Input: part model. Units: mm. Frame: model coordinates. A direction names the side the tool comes from. Coordinates: 2 decimals unless noted, no trailing zeros. Loops run counter-clockwise (first coordinate to the right, second up) from the corner with the lowest first, then second, coordinate; pieces in that order, holes last.
(1) Section C-C, the plane y = 21. Return loops of the section in (x, z), then the cut area to 3 significant figures.
(2) Set-up query: faces 5 (the face through (0.75, 43.7, -0.1)), 6 (the face through (1, 44, -17)), 7 (the face through (-1.2, 47.5, 0.1)). Return all of +Z, -Z, +X, -X, +Y, -Y with unobstructed straight access to the full face (end or side cutting, diameter ignored); none if empty.
(3) Section B-B, the plane z = -10.5. Return loops of the section in (x, y).
(4) Section A-A, the plane z = 0. Return loops of the section in (x, y), then the cut area to 3 significant figures.
(5) Contact query for flat-ended pins moving along their axis: P1, Ø12, axis at y = 27, z = -19.5, coming from the -X side; P2, Ø1.1, axis at x = 1, z = 8, coming from the +Y side; P3, Ø0.5, axis at x = -1.5, z = 2, coming from the +Y side; P4, Ø0.8, axis at x = 1, z = -1, coming from the +Y side. Output: stop coordinate, or through.
(6) Mould query, pull axis Z, two halves, no side actions, for faces 1 (the face through (0, -1, -28.25)), 2 (the face through (1.3, 47.5, 0.1)), 3 (the face through (-0.75, 43.7, -0.1)), 4 (the face through (1, 44, 16)). Classes: released by +Z, released by -Z, zero draft, split by the parting line, or undercut.
(7) Line query: L1, parallel to Z at x = 0.3, y = 23; L2, parallel to Z at x = -1.05, y = 31; L3, parallel to Y at x = 0.9, z = 8. Output: solid intervals per line, ascending.
```python
from build123d import *

# Parameters (mm, degrees)
F1_DEPTH      = 1.75
F2_W          = 1.5
F2_H          = 55
F3_DEPTH      = 43.25
F3_DEPTH_BACK = 58.6


with BuildPart() as f1:
    # F0 (on Right) → F1 (new body, symmetric)
    with BuildSketch(Plane.YZ):
        Polygon((-42.75, -27), (-42.75, 27), (-41.75, 27), (-41.75, 28.25), (-44, 28.25), (-44, -28.25), (-41.75, -28.25), (-41.75, -27), align=None)
        Polygon((-41.75, 27), (-42.75, 27), (-42.75, -27), (-41.75, -27), (-41.75, -26), (-41.75, 26), align=None)
        Polygon((-41.75, 28.25), (-41.75, 27), (42.75, 27), (42.75, -27), (-41.75, -27), (-41.75, -28.25), (44, -28.25), (44, -5), (44, -3.5), (44, 3.5), (44, 5), (44, 28.25), align=None)
        with BuildLine():
            ThreePointArc((44, -5), (49, 0), (44, 5))
            Line((44, 5), (44, 3.5))
            ThreePointArc((44, 3.5), (47.5, 0), (44, -3.5))
            Line((44, -3.5), (44, -5))
        make_face()
    extrude(amount=F1_DEPTH, both=True)

    # F2 (on Front) → F3 (cut, two sides)
    with BuildSketch(Plane.XZ) as f3_sk:
        Rectangle(F2_W, F2_H)
    extrude(amount=F3_DEPTH, mode=Mode.SUBTRACT)
    extrude(f3_sk.sketch, amount=-F3_DEPTH_BACK, mode=Mode.SUBTRACT)


solid = f1.part
```
Report:
1. outline: (-1.75, -28.25) - (1.75, -28.25) - (1.75, -27) - (0.75, -27) - (0.75, -27.5) - (-0.75, -27.5) - (-0.75, -27) - (-1.75, -27) - close; (-1.75, 27) - (-0.75, 27) - (-0.75, 27.5) - (0.75, 27.5) - (0.75, 27) - (1.75, 27) - (1.75, 28.25) - (-1.75, 28.25) - close
1. area: 7.25 mm2
2. face 5: +Y
2. face 6: -Z, +X, -X, +Y
2. face 7: +X, -X
3. outline: (-1.75, -44) - (1.75, -44) - (1.75, -41.75) - (0.75, -41.75) - (0.75, -43.25) - (-0.75, -43.25) - (-0.75, -41.75) - (-1.75, -41.75) - close; (-1.75, 42.75) - (-0.75, 42.75) - (-0.75, 44) - (-1.75, 44) - close; (0.75, 42.75) - (1.75, 42.75) - (1.75, 44) - (0.75, 44) - close
4. outline: (-1.75, -44) - (1.75, -44) - (1.75, -41.75) - (0.75, -41.75) - (0.75, -43.25) - (-0.75, -43.25) - (-0.75, -41.75) - (-1.75, -41.75) - close; (-1.75, 42.75) - (-0.75, 42.75) - (-0.75, 44) - (-1.75, 44) - close; (-1.75, 47.5) - (-0.75, 47.5) - (-0.75, 49) - (-1.75, 49) - close; (0.75, 42.75) - (1.75, 42.75) - (1.75, 44) - (0.75, 44) - close; (0.75, 47.5) - (1.75, 47.5) - (1.75, 49) - (0.75, 49) - close
4. area: 11.1 mm2
5. P1: passes through
5. P2: stops at y = 44
5. P3: stops at y = 48.68
5. P4: stops at y = 48.96
6. face 1: released by -Z
6. face 2: undercut
6. face 3: undercut
6. face 4: zero draft
7. L1: z = -28.25 to -27.5, 27.5 to 28.25
7. L2: z = -28.25 to -27, 27 to 28.25
7. L3: y = -44 to -41.75, 42.75 to 44
